Geometry: see drawing. Coordinates: mm, zero at the bounding-box minimum. A direction names the side the tool comes from. Round coordinates to 2 decimals unless told otherwise and drop trailing zeros. Order: outer loops, then holes, each group sorted by start corner. A loop starts at its lowest first (then second) coordinate and runs counter-clockwise, first axis right, second up.
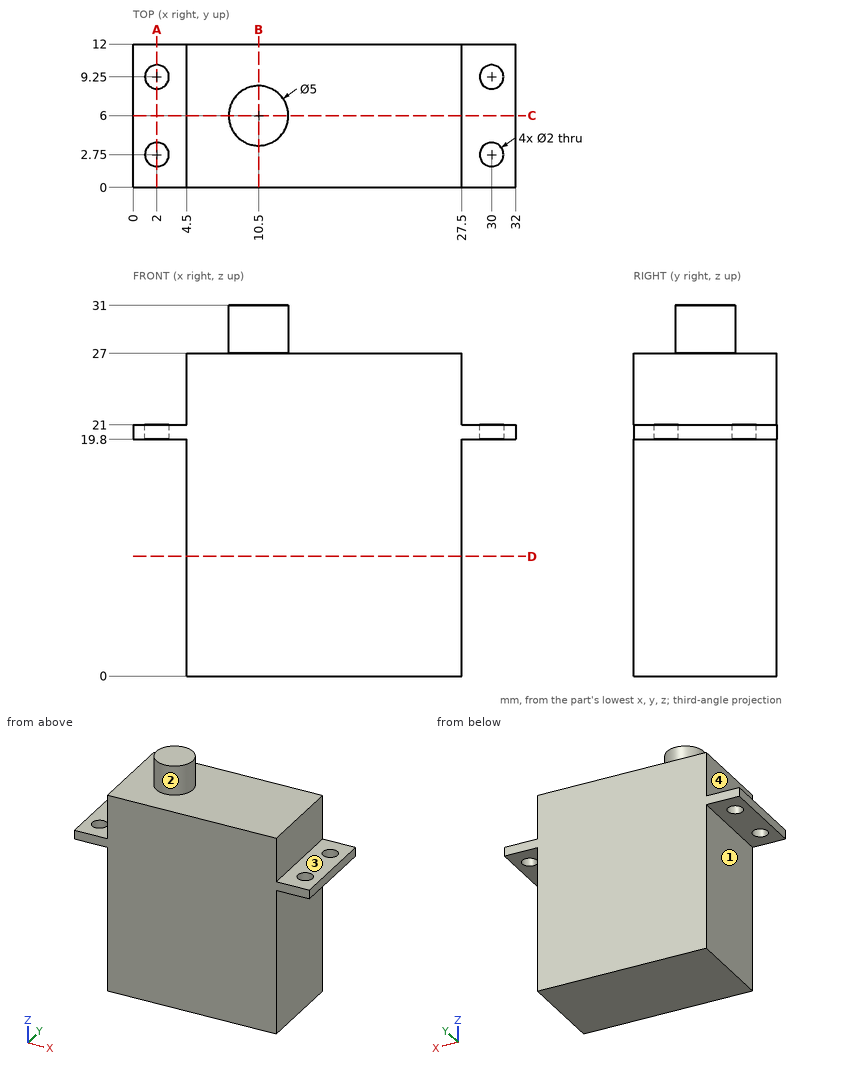
1. Access query for the marked faces 1, 2, 3 and 4. Directions: +Z, -Z, +X, -X, +Y, -Y. A direction counts if a zero-diameter tool reaches every point of the face in a straight line with its end or side. Return the directions, or none.
2. Section C-C on y = 6. Return loops of the section in (x, z).
3. First-contact query: pin 1 (4 mm diameter, centred on y = 7, z = 12.5, fed in from -X); pin 2 (3 mm diameter, centred on y = 5, z = 23.5, fed in from +X); pin 3 (3 mm diameter, centred on x = 5.5, z = 6, fed in from -Y); pin 4 (1 mm diameter, centred on x = 19, y = 9, fed in from +Z). Flat tips, straight axial feed; report the tip coordinate or a pass-through.
4. Section B-B on x = 10.5. Return loops of the section in (y, z), plus the area to 3 significant figures.
5. Section A-A on x = 2. Return loops of the section in (y, z).
6. Section D-D on z = 10. Return loops of the section in (x, y).
7. Line query: line 1 along Y through (x, z) = (30, 20.15); line 2 along X through (y, z) = (7.5, 12); line 3 along Z through (x, y) = (4, 8). Output: solid intervals per line, ascending.
Result:
1. face 1: -Z, -X, +Y, -Y
1. face 2: +Z
1. face 3: +Z, +X, +Y, -Y
1. face 4: +Z, -X, +Y, -Y
2. outline: (0, 19.8) - (4.5, 19.8) - (4.5, 0) - (27.5, 0) - (27.5, 19.8) - (32, 19.8) - (32, 21) - (27.5, 21) - (27.5, 27) - (13, 27) - (13, 31) - (8, 31) - (8, 27) - (4.5, 27) - (4.5, 21) - (0, 21) - close
3. pin 1: stops at x = 4.5
3. pin 2: stops at x = 27.5
3. pin 3: stops at y = 0
3. pin 4: stops at z = 27
4. outline: (0, 0) - (12, 0) - (12, 27) - (8.5, 27) - (8.5, 31) - (3.5, 31) - (3.5, 27) - (0, 27) - close
4. area: 344 mm2
5. outline: (0, 19.8) - (1.75, 19.8) - (1.75, 21) - (0, 21) - close; (3.75, 19.8) - (8.25, 19.8) - (8.25, 21) - (3.75, 21) - close; (10.25, 19.8) - (12, 19.8) - (12, 21) - (10.25, 21) - close
6. outline: (4.5, 0) - (27.5, 0) - (27.5, 12) - (4.5, 12) - close
7. line 1: y = 0 to 1.75, 3.75 to 8.25, 10.25 to 12
7. line 2: x = 4.5 to 27.5
7. line 3: z = 19.8 to 21
